Work out the finished part from the listing and answer in its coordinate system (mm). A direction names the side the tool comes from. Coordinates: 2 decimals unless noted, no trailing zeros. Order: outer loops, then holes, each group sorted by start corner. A loop starts at its lowest first (then second) coordinate and runs counter-clockwise, first axis right, second up. Notation, with made-up numbers: M -23,-33 L 28,-33 A21 cw 28,0 Z; hole C 9.25,-38.75 d3. An arc over 180 degrees is marked long. Answer in a Markdown table with one row per item. Add a question column.
Item 1: The part is cut by section D-D (y = 3.05). Write down the section's boundary in (x, z) (3 decimals).
Item 2: Flat-ended cylindrical pins translate along their axes: pin 1 Ø1 at (x, y) = (-1, 3) entering from +Z; pin 2 Ø2 at (y, z) = (3.5, -3) entering from -X; pin 3 Ø0.8 at (y, z) = (2, -8.5) entering from -X. Find the tip coordinate at first contact, or state that the pin passes through.
Item 3: Consider line 1 (X direction, y = 2.2, z = -25); line 2 (X direction, y = 2.5, z = -13); line 3 (Y direction, x = -1.75, z = 2). Determine where each line is inside the solid, lowest interval first. Write a range as from..to.
Item 4: The part is cut by section C-C (z = -14). Write down the section's boundary in (x, y).
Item 5: The part is cut by section B-B (y = 1.75). Write down the section's boundary in (x, z) (3 decimals).
Item 6: The mould has two halves that part along Z. Classify faces 1 (the face through (0, 0, -12)), 2 (the face through (0, 2, -26)), 3 (the face through (0.08, 1.97, -28.75)): released by +Z, released by -Z, zero draft, split by the parting line, or undercut.
Item 7: The part is cut by section A-A (x = 0). Write down the section's boundary in (y, z), then the cut area to 3 significant figures.
Item 8: Which of the six approach directions +Z, -Z, +X, -X, +Y, -Y give full straight-line access (tool end or side, diameter ignored) to faces 4 (the face through (0, 3, -1.1)), 5 (the face through (-2.706, 1.356, 0.894)), 6 (the face through (0, 4, -12))?
from build123d import *

# Parameters (mm, degrees)
SKETCH1_R           = 1
BOSS_EXTRUDE1_DEPTH = 4
CUT_EXTRUDE1_DEPTH  = 2.75
CUT_EXTRUDE4_DEPTH  = 10


with BuildPart() as part:
    # Sketch1 → Boss-Extrude1 (new body)
    with BuildSketch(Plane(origin=(0, 0, 0), x_dir=(1, 0, 0), z_dir=(0, 1, 0))):
        with BuildLine():
            Line((4.249149915, 0.085), (3.749249925, 25.075))
            ThreePointArc((3.749249925, 25.075), (0, 28.75), (-3.749249925, 25.075))
            Line((-3.749249925, 25.075), (-4.249149915, 0.085))
            ThreePointArc((-4.249149915, 0.085), (0, -4.25), (4.249149915, 0.085))
        make_face()
        with Locations(Location((0, 25, 0), (0, 0, 270))):
            Circle(SKETCH1_R, mode=Mode.SUBTRACT)
    extrude(amount=BOSS_EXTRUDE1_DEPTH)

    # Sketch2 → Cut-Extrude1 (cut)
    with BuildSketch(Plane(origin=(0, 0, 0), x_dir=(1, 0, 0), z_dir=(0, 1, 0))):
        with BuildLine():
            Line((2.15, 15), (2.15, 1.870828693))
            ThreePointArc((2.15, 1.870828693), (-2.669269563, -0.998749218), (2.85, 0))
            Line((2.85, 0), (2.85, 15))
            Line((2.85, 15), (2.15, 15))
        make_face()
    extrude(amount=CUT_EXTRUDE1_DEPTH, mode=Mode.SUBTRACT)

    # Sketch4 → Cut-Extrude4 (cut)
    with BuildSketch(Plane.XZ.offset(-2.75)):
        with BuildLine():
            Line((1.459053249, 1.440022089), (1.447376313, 1.451758179))
            ThreePointArc((1.447376313, 1.451758179), (-0.785932109, 1.893359638), (-2.05, 0))
            Line((-2.05, 0), (2.05, 0))
            ThreePointArc((2.05, 0), (1.896517751, 0.778280425), (1.459053249, 1.440022089))
        make_face()
        with BuildLine():
            Line((2.05, 0), (-2.05, 0))
            ThreePointArc((-2.05, 0), (-1.968344863, -0.572816289), (-1.729884389, -1.1))
            Line((-1.729884389, -1.1), (1.729884389, -1.1))
            ThreePointArc((1.729884389, -1.1), (1.968344863, -0.572816289), (2.05, 0))
        make_face()
    extrude(amount=-CUT_EXTRUDE4_DEPTH, mode=Mode.SUBTRACT)


solid = part.part
Reply:
| question | item | result |
|---|---|---|
| 1 | outline | M -4.249,-0.085 L -3.749,-25.075 A3.75 ccw 3.749,-25.075 L 4.249,-0.085 A4.25 ccw long Z; hole M -1.73,-1.1 L 1.73,-1.1 A2.05 ccw 1.459,1.44 L 1.447,1.452 A2.05 ccw Z; hole C 0,-25 d2 |
| 2 | pin 1 | stops at z = 4.22 |
| 2 | pin 2 | stops at x = -4.21 |
| 2 | pin 3 | stops at x = -4.09 |
| 3 | line 1 | x = -3.75..-1, 1..3.75 |
| 3 | line 2 | x = -3.99..2.15, 2.85..3.99 |
| 3 | line 3 | y = 2.75..4 |
| 4 | outline | M -3.97,0 L 2.15,0 L 2.15,2.75 L 2.85,2.75 L 2.85,0 L 3.97,0 L 3.97,4 L -3.97,4 Z |
| 5 | outline | M -4.249,-0.085 L -3.749,-25.075 A3.75 ccw 3.749,-25.075 L 4.249,-0.085 A4.25 ccw long Z; hole C 0,-25 d2; hole M 2.15,-15 L 2.85,-15 L 2.85,0 A2.85 ccw long 2.15,-1.871 Z |
| 6 | face 1 | zero draft |
| 6 | face 2 | undercut |
| 6 | face 3 | released by -Z |
| 7 | outline | M 0,-28.75 L 4,-28.75 L 4,-26 L 0,-26 Z; M 0,-24 L 4,-24 L 4,-1.1 L 2.75,-1.1 L 2.75,-2.85 L 0,-2.85 Z; M 0,2.85 L 2.75,2.85 L 2.75,2.05 L 4,2.05 L 4,4.25 L 0,4.25 Z |
| 7 | area | 104 mm2 |
| 8 | face 4 | +Y, -Y |
| 8 | face 5 | -Y |
| 8 | face 6 | +Z, -Z, +X, -X, +Y |
